```python
from build123d import *

# Parameters (mm, degrees)
BOX024_W                  = 115
BOX024_H                  = 115
BOX024_DEPTH              = 2
BOX023_W                  = 115
BOX023_H                  = 115
BOX023_DEPTH              = 60
BOX022_W                  = 20
BOX022_H                  = 165
BOX022_DEPTH              = 165
BOX025_W                  = 9
BOX025_H                  = 3
BOX025_DEPTH              = 30
BOX026_W                  = 9
BOX026_H                  = 3
BOX026_DEPTH              = 30
BOX021_W                  = 115
BOX021_H                  = 115
BOX021_DEPTH              = 60
BOX020_W                  = 165
BOX020_H                  = 165
BOX020_DEPTH              = 15
CUT006_PLACEMENT_ANGLE    = 90
BOX027_W                  = 12
BOX027_H                  = 5
BOX027_DEPTH              = 40
FUSION003_PLACEMENT_ANGLE = 90


with BuildPart() as cube019:
    # Box024 → Box024 (new body)
    with BuildSketch(Plane(origin=(129, -57, 61), x_dir=(0, 0, 1), z_dir=(-1, 0, 0))):
        with Locations((57.5, 57.5)):
            Rectangle(BOX024_W, BOX024_H)
    extrude(amount=BOX024_DEPTH)


with BuildPart() as cube018:
    # Box023 → Box023 (new body)
    with BuildSketch(Plane(origin=(149, -57, 61), x_dir=(0, 0, 1), z_dir=(-1, 0, 0))):
        with Locations((57.5, 57.5)):
            Rectangle(BOX023_W, BOX023_H)
    extrude(amount=BOX023_DEPTH)


with BuildPart() as cut007:
    # Box022 → Box022 (new body)
    with BuildSketch(Plane(origin=(109, -82, 38), x_dir=(1, 0, 0), z_dir=(0, 0, 1))):
        with Locations((10, 82.5)):
            Rectangle(BOX022_W, BOX022_H)
    extrude(amount=BOX022_DEPTH)

    # Cut007: cut Cube018
    add(cube018.part, mode=Mode.SUBTRACT)


with BuildPart() as cube020:
    # Box025 → Box025 (new body)
    with BuildSketch(Plane(origin=(105, -60, 140), x_dir=(1, 0, 0), z_dir=(0, 0, 1))):
        with Locations((4.5, 1.5)):
            Rectangle(BOX025_W, BOX025_H)
    extrude(amount=BOX025_DEPTH)


with BuildPart() as cube021:
    # Box026 → Box026 (new body)
    with BuildSketch(Plane(origin=(105, 58, 140), x_dir=(1, 0, 0), z_dir=(0, 0, 1))):
        with Locations((4.5, 1.5)):
            Rectangle(BOX026_W, BOX026_H)
    extrude(amount=BOX026_DEPTH)


with BuildPart() as cube016:
    # Box021 → Box021 (new body)
    with BuildSketch(Plane(origin=(25, 25, -7), x_dir=(1, 0, 0), z_dir=(0, 0, 1))):
        with Locations((57.5, 57.5)):
            Rectangle(BOX021_W, BOX021_H)
    extrude(amount=BOX021_DEPTH)


with BuildPart() as bellows001:
    # Box020 → Box020 (new body)
    with BuildSketch(Plane.XY):
        with Locations((82.5, 82.5)):
            Rectangle(BOX020_W, BOX020_H)
    extrude(amount=BOX020_DEPTH)

    # Cut006: cut Cube016
    add(cube016.part, mode=Mode.SUBTRACT)


with BuildPart() as bellows001_1:
    # Cut006 placement: moved
    add(bellows001.part.moved(Location((144, -82, 36))).rotate(Axis((144, -82, 36), (0, -1, 0)), CUT006_PLACEMENT_ANGLE))


with BuildPart() as ground_glass:
    # Box027 → Box027 (new body)
    with BuildSketch(Plane(origin=(122, 81, 138), x_dir=(1, 0, 0), z_dir=(0, 0, 1))):
        with Locations((6, 2.5)):
            Rectangle(BOX027_W, BOX027_H)
    extrude(amount=BOX027_DEPTH)

    # Fusion003: union Cube019, Cut007, Cube020, Cube021, bellows001
    add(cube019.part)
    add(cut007.part)
    add(cube020.part)
    add(cube021.part)
    add(bellows001_1.part)


with BuildPart() as ground_glass_1:
    # Fusion003 placement: moved
    add(ground_glass.part.moved(Location((84.5, 551, -34))).rotate(Axis((84.5, 551, -34), (0, 0, -1)), FUSION003_PLACEMENT_ANGLE))


solid = ground_glass_1.part
```
The model under review builds one solid part; all positions refer to its coordinate system, in mm. A direction names the side the tool comes from. Round coordinates to 2 decimals unless told otherwise and drop trailing zeros. Write each loop counter-clockwise with the first axis right and the second up, starting at its lowest first coordinate (ties: lowest second). Pieces come first, ordered by that corner, then holes. Notation, with made-up numbers: (-28, 81) - (-14, 81) arc R15 cw to (-14, 91) - close; hole circle Ø6 at (-24.5, 75.25). An arc over 180 degrees is marked (long way). One line per question, with ' | ' between items.
Item 1: Add section C-C, the plane x = 118. Give the boundary of the cut face in (y, z), then the cut area to 3 significant figures.
Resolved:
outline: (407, 2) - (422, 2) - (422, 4) - (442, 4) - (442, 27) - (424, 27) - (424, 142) - (442, 142) - (442, 169) - (422, 169) - (422, 167) - (407, 167) - (407, 142) - (422, 142) - (422, 27) - (407, 27) - close | area: 1,980 mm2
Item 2: Add section B-B, the plane z = 130. Give the boundary of the cut face in (x, y).
Resolved:
outline: (2.5, 407) - (27.5, 407) - (27.5, 422) - (142.5, 422) - (142.5, 407) - (167.5, 407) - (167.5, 417) - (170.5, 417) - (170.5, 429) - (167.5, 429) - (167.5, 442) - (145.5, 442) - (145.5, 446) - (142.5, 446) - (142.5, 424) - (27.5, 424) - (27.5, 446) - (24.5, 446) - (24.5, 442) - (2.5, 442) - close
Item 3: Add section D-D, the plane y = 434.5. Give the boundary of the cut face in (x, z), then the cut area to 3 significant figures.
Resolved:
outline: (2.5, 4) - (167.5, 4) - (167.5, 169) - (2.5, 169) - close; hole (27.5, 27) - (142.5, 27) - (142.5, 142) - (27.5, 142) - close | area: 14,000 mm2
Item 4: Add section A-A, the plane y = 419.5. Give the boundary of the cut face in (x, z), then the cut area to 3 significant figures.
Resolved:
outline: (2.5, 2) - (167.5, 2) - (167.5, 104) - (170.5, 104) - (170.5, 144) - (167.5, 144) - (167.5, 167) - (2.5, 167) - close; hole (27.5, 27) - (142.5, 27) - (142.5, 142) - (27.5, 142) - close | area: 14,100 mm2
Item 5: To check wall thickness, follow probe 1 along X at (y, z) = (434.5, 108); probe 2 along Z at (x, y) = (104.5, 432); probe 3 along Z at (x, y) = (50.5, 412). State the ranges of each line that lie inside material, in increasing order.
Resolved:
probe 1: x = 2.5 to 27.5, 142.5 to 167.5 | probe 2: z = 4 to 27, 142 to 169 | probe 3: z = 2 to 27, 142 to 167
Item 6: The part is to be moulded in two halves that separate along X. For faces 1 (the face through (86, 407, 10)), 2 (the face through (84, 433, 27)), 3 (the face through (2.5, 424, 84)), say which applies: pulls with the +X half, pulls with the -X half, needs draft (parallel to the pull), parting line crosses it, or undercut.
Resolved:
face 1: needs draft | face 2: undercut | face 3: pulls with the -X half
Item 7: For faces 4 (the face through (142.5, 414, 84)), 5 (the face through (84, 414, 167)), 6 (the face through (86, 424, 84)), 7 (the face through (86, 432, 4)), 8 (the face through (145.5, 444, 121)), list the 3-axis set-ups (+Z, -Z, +X, -X, +Y, -Y) from which the entire face can be reached by the end or side of a thin tool; tool diameter is ignored.
Resolved:
face 4: -Y | face 5: +Z, +X, -X, -Y | face 6: +Y | face 7: -Z, +X, -X, +Y | face 8: +Z, -Z, +X, +Y
Item 8: For P1, Ø12, axis at y = 411.5, z = 109, coming from the +X side; P2, Ø10, axis at x = 78.5, z = 28, coming from the +Y side; P3, Ø6, axis at x = 115.5, y = 434.5, coming from the -Z side; P4, Ø6, axis at x = 80.5, y = 414.5, coming from the +Z side, all flat-tipped, find the tip position at first contact; note any pin that passes through.
Resolved:
P1: stops at x = 170.5 | P2: stops at y = 442 | P3: stops at z = 4 | P4: stops at z = 167
